Geometry: see drawing. Coordinates: mm, zero at the bounding-box minimum. Give positions to 0.01 mm unless a question says otherwise; leave off trailing zeros. Loops run counter-clockwise (first coordinate to the right, second up) from the corner with the lowest first, then second, coordinate; pieces in that order, holes last. Notation, with made-up numbers: (-1.5, 64) -> (2.5, 64) arc R8 cw to (2.5, 79) -> close; hole circle Ø7 at (-37, 71.5). An arc over 180 degrees is marked (long way). Return JSON: item names as keys, results as strings. Group by question number.
(1) Cut plane A-A on x = 19. Return loops of the section in (y, z), then the cut area to 3 significant figures.
(2) Cut plane B-B on z = 7.5. Return loops of the section in (x, y), then the cut area to 3 significant figures.
(3) Cut plane C-C on x = 26.5. Return loops of the section in (y, z), then the cut area to 3 significant figures.
(4) Draft query along X for the marked faces 1, 2, 3 and 4. Return one class per face: released by +X, released by -X, zero draft, split by the parting line, or undercut.
(5) Ray query, line 1 (Z direction, x = 19, y = 10.7); line 2 (Y direction, x = 33.5, z = 25); line 3 (Z direction, x = 35, y = 5.5) (1 decimal). Return the intervals inside material, ascending. Write a range as from..to.
(6) Pin query (flat end, axial travel): pin 1 (9 mm diameter, centred on x = 19, z = 20.5, fed in from -Y). Return the tip coordinate at first contact, or that it passes through.
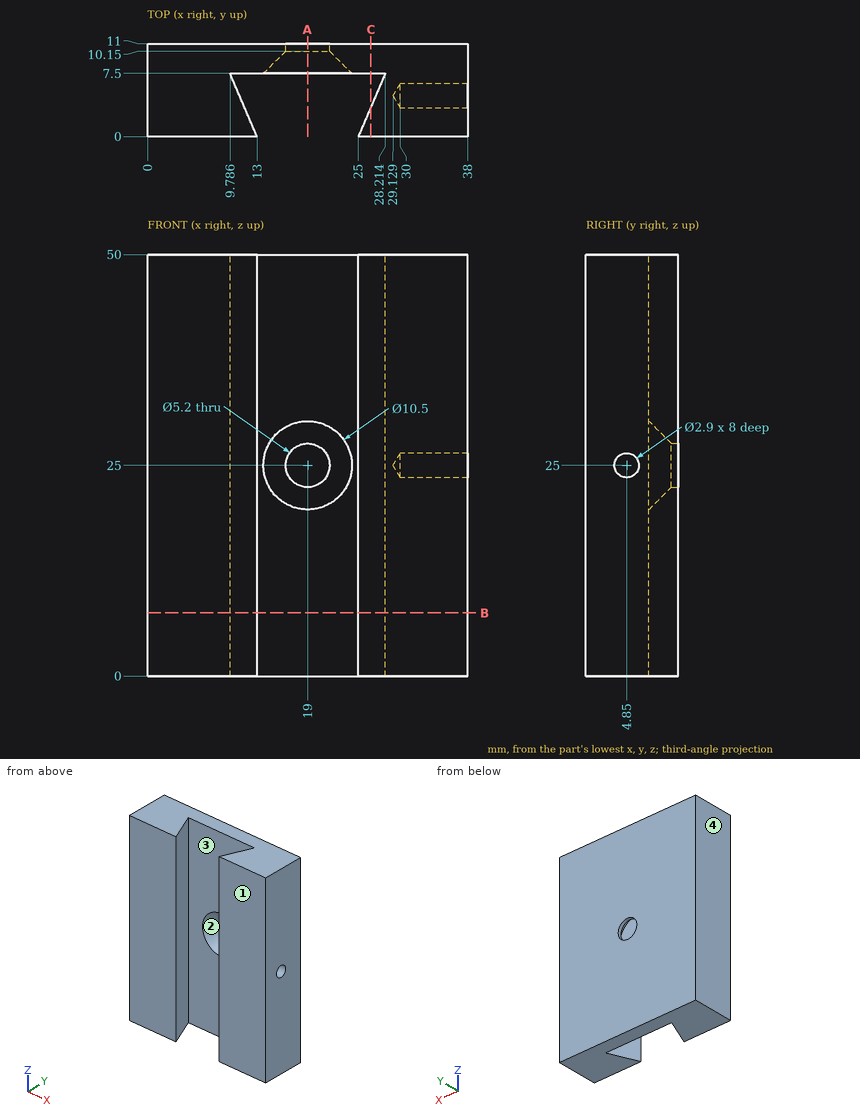
Answers:
{
 "1": {"outline": "(7.5, 0) -> (11, 0) -> (11, 22.4) -> (10.15, 22.4) -> (7.5, 19.75) -> close; (7.5, 30.25) -> (10.15, 27.6) -> (11, 27.6) -> (11, 50) -> (7.5, 50) -> close", "area": "150 mm²"},
 "2": {"outline": "(0, 0) -> (13, 0) -> (9.79, 7.5) -> (28.21, 7.5) -> (25, 0) -> (38, 0) -> (38, 11) -> (0, 11) -> close", "area": "304 mm²"},
 "3": {"outline": "(0, 0) -> (3.5, 0) -> (3.5, 50) -> (0, 50) -> close; (7.5, 0) -> (11, 0) -> (11, 50) -> (7.5, 50) -> close", "area": "350 mm²"},
 "4": {"face 1": "zero draft", "face 2": "undercut", "face 3": "undercut", "face 4": "released by -X"},
 "5": {"line 1": "0..22.4, 27.6..50", "line 2": "0..3.4, 6.3..11", "line 3": "0..23.7, 26.3..50"},
 "6": {"pin 1": "y = 7.5"}
}
